from build123d import *

# Parameters (mm, degrees)
SKETCH1_R           = 31
BOSS_EXTRUDE1_DEPTH = 8
SKETCH2_R           = 20
BOSS_EXTRUDE2_DEPTH = 51
SKETCH3_R           = 12.5
CUT_EXTRUDE1_DEPTH  = 74.505101864
SKETCH4_R           = 4.6
CUT_EXTRUDE2_DEPTH  = 5.4
SKETCH5_R           = 2.75
CUT_EXTRUDE3_DEPTH  = 70.245649683


with BuildPart() as part:
    # Sketch1 → Boss-Extrude1 (new body)
    with BuildSketch(Plane(origin=(0, 0, 0), x_dir=(1, 0, 0), z_dir=(0, 1, 0))):
        with Locations(Location((0, 0, 0), (0, 0, 270))):
            Circle(SKETCH1_R)
    extrude(amount=BOSS_EXTRUDE1_DEPTH)

    # Sketch2 → Boss-Extrude2 (add)
    with BuildSketch(Plane(origin=(0, 8, 0), x_dir=(1, 0, 0), z_dir=(0, 1, 0))):
        with Locations(Location((0, 0, 0), (0, 0, 270))):
            Circle(SKETCH2_R)
    extrude(amount=BOSS_EXTRUDE2_DEPTH)

    # Sketch3 → Cut-Extrude1 (cut, through all)
    with BuildSketch(Plane(origin=(0, 59, 0), x_dir=(1, 0, 0), z_dir=(0, 1, 0))):
        with Locations(Location((0, 0, 0), (0, 0, 270))):
            Circle(SKETCH3_R)
    extrude(amount=-CUT_EXTRUDE1_DEPTH, mode=Mode.SUBTRACT)

    # Sketch4 → Cut-Extrude2 (cut)
    with BuildSketch(Plane.XZ):
        with Locations(Location((0, -25.5, 0), (0, 0, 270))):
            Circle(SKETCH4_R)
        with Locations(Location((-25.5, 0, 0), (0, 0, 270))):
            Circle(SKETCH4_R)
        with Locations(Location((0, 25.5, 0), (0, 0, 270))):
            Circle(SKETCH4_R)
        with Locations(Location((25.5, 0, 0), (0, 0, 270))):
            Circle(SKETCH4_R)
    extrude(amount=-CUT_EXTRUDE2_DEPTH, mode=Mode.SUBTRACT)

    # Sketch5 → Cut-Extrude3 (cut, through all)
    with BuildSketch(Plane.XZ.offset(-5.4)):
        with Locations(Location((25.5, 0, 0), (0, 0, 270))):
            Circle(SKETCH5_R)
        with Locations(Location((0, -25.5, 0), (0, 0, 270))):
            Circle(SKETCH5_R)
        with Locations(Location((-25.5, 0, 0), (0, 0, 270))):
            Circle(SKETCH5_R)
        with Locations(Location((0, 25.5, 0), (0, 0, 270))):
            Circle(SKETCH5_R)
    extrude(amount=-CUT_EXTRUDE3_DEPTH, mode=Mode.SUBTRACT)


solid = part.part
Here's how the part is built. I have some questions about the finished solid (model axes, mm). A direction names the side the tool comes from. Coordinates: 2 decimals unless noted, no trailing zeros. Write each loop counter-clockwise with the first axis right and the second up, starting at its lowest first coordinate (ties: lowest second). Pieces come first, ordered by that corner, then holes.
1) If we section it at A-A (z = 0): List the corners of the cut face in (x, y) for me.
Filled in:
outline: (-31, 0) - (-30.1, 0) - (-30.1, 5.4) - (-28.25, 5.4) - (-28.25, 8) - (-31, 8) - close; (-22.75, 5.4) - (-20.9, 5.4) - (-20.9, 0) - (-12.5, 0) - (-12.5, 59) - (-20, 59) - (-20, 8) - (-22.75, 8) - close; (12.5, 0) - (20.9, 0) - (20.9, 5.4) - (22.75, 5.4) - (22.75, 8) - (20, 8) - (20, 59) - (12.5, 59) - close; (28.25, 5.4) - (30.1, 5.4) - (30.1, 0) - (31, 0) - (31, 8) - (28.25, 8) - close
2) Which directions (+Z, -Z, +X, -X, +Y, -Y) give clear straight access to the entire face, cutting with the end or side of a thin tool? Please do faces 1 (the face through (-2.8, 2.66, 29.15)), 2 (the face through (28.227, 6.682, 0.358)), 3 (the face through (0.4, 8, 20.2)).
Filled in:
face 1: -Y
face 2: +Y, -Y
face 3: +Y
3) I'm going to push flat-ended pins straight in: pin 1 (8.5 mm diameter, centred on x = -25.5, z = 0, fed in from -Y); pin 2 (12 mm diameter, centred on x = -17.5, z = -6, fed in from -Y); pin 3 (1.5 mm diameter, centred on y = 48.5, z = 15, fed in from -X); pin 4 (5 mm diameter, centred on y = 25, z = 0, fed in from -X). Where does each tip first touch, or does it pass through?
Filled in:
pin 1: stops at y = 5.4
pin 2: stops at y = 0
pin 3: stops at x = -14.03
pin 4: stops at x = -20
4) If we section it at B-B (x = 0): List the corners of the cut face in (y, z) for me, plus the area to 3 significant figures.
Filled in:
outline: (0, -31) - (8, -31) - (8, -28.25) - (5.4, -28.25) - (5.4, -30.1) - (0, -30.1) - close; (0, -20.9) - (5.4, -20.9) - (5.4, -22.75) - (8, -22.75) - (8, -20) - (59, -20) - (59, -12.5) - (0, -12.5) - close; (0, 12.5) - (59, 12.5) - (59, 20) - (8, 20) - (8, 22.75) - (5.4, 22.75) - (5.4, 20.9) - (0, 20.9) - close; (0, 30.1) - (5.4, 30.1) - (5.4, 28.25) - (8, 28.25) - (8, 31) - (0, 31) - close
area: 933 mm2
5) If I drill on line 1 (X direction, y = 2.15, z = 0); line 2 (X direction, y = 6.7, z = 0); line 3 (Y direction, x = -24, z = -4.5), over which ranges is the centre line in solid material (lowest first)?
Filled in:
line 1: x = -31 to -30.1, -20.9 to -12.5, 12.5 to 20.9, 30.1 to 31
line 2: x = -31 to -28.25, -22.75 to -12.5, 12.5 to 22.75, 28.25 to 31
line 3: y = 0 to 8
6) If we section it at D-D (y = 25.5): List the corners of the cut face in (x, z) for me.
Filled in:
outline: circle Ø40 at (0, 0); hole circle Ø25 at (0, 0)
7) Thinking about a two-plate mould opening in X: for faces 4 (the face through (0, 0, 13)), 5 (the face through (-19.524, 33.143, -4.336)), 6 (the face through (0.121, 6.682, -22.753)), which applies, +X half, -X half, draft (parallel to the pull), parting line (faces both ways), or undercut?
Filled in:
face 4: draft
face 5: parting line
face 6: undercut
8) If we section it at C-C (z = 10): List the corners of the cut face in (x, y) for me.
Filled in:
outline: (-29.34, 0) - (-7.5, 0) - (-7.5, 59) - (-17.32, 59) - (-17.32, 8) - (-29.34, 8) - close; (7.5, 0) - (29.34, 0) - (29.34, 8) - (17.32, 8) - (17.32, 59) - (7.5, 59) - close
